from build123d import *

# Parameters (mm, degrees)
F1_DEPTH = 6.35


with BuildPart() as f1:
    # F0 (on Front) → F1 (new body)
    with BuildSketch(Plane.XZ):
        with BuildLine():
            Line((147.03905, 56.8491), (26.060874, 15.470934))
            ThreePointArc((26.060874, 15.470934), (14.468308, -7.009272), (35.415419, -21.185511))
            Line((35.415419, -21.185511), (159.893201, -17.296974))
            ThreePointArc((159.893201, -17.296974), (196.909173, 27.30746), (147.03905, 56.8491))
        make_face()
        with BuildLine():
            ThreePointArc((28.604817, 5.287778), (30.133109, 5.973494), (31.764223, 6.354742))
            Line((31.764223, 6.354742), (41.633012, -1.638817))
            ThreePointArc((41.633012, -1.638817), (40.945432, -5.75352), (38.427272, -9.079542))
            Line((38.427272, -9.079542), (28.954331, -10.074033))
            ThreePointArc((28.954331, -10.074033), (24.867546, -5.657956), (24.608037, 0.353383))
            Line((24.608037, 0.353383), (28.604817, 5.287778))
        make_face(mode=Mode.SUBTRACT)
    extrude(amount=F1_DEPTH)


solid = f1.part
Read the model definition and answer for the solid it produces. Units are mm, in the model's axes. A direction names the side the tool comes from. Give positions to 0.01 mm unless a question says otherwise; leave off trailing zeros. Write each loop counter-clockwise with the first axis right and the second up, starting at its lowest first coordinate (ties: lowest second). Pieces come first, ordered by that corner, then holes. Notation, with made-up numbers: (16, 69) - (42, 69) arc R20 ccw to (42, 91) - close; hole circle Ø4 at (55, 46.5). An arc over 180 degrees is marked (long way). Use CSV: the item, a comma, the result in double quotes. Start each with the question number.
Item 1: The mould has two halves that part along Z. Classify faces 3 (the cylindrical face through (24.901, -3.131, -5.737)), 4 (the cylindrical face through (14.376, -3.131, -6.633)), 5 (the flat face through (104, 0, 10)): pulls with the +Z half, pulls with the -Z half, needs draft (parallel to the pull), parting line crosses it, or undercut.
Item 2: The part is cut by section B-B, the plane z = -4. Give the vertices of the cut face in (x, y).
Item 3: The part is cut by section C-C, the plane x = 97.5. Give the vertices of the cut face in (y, z).
Item 4: The part is cut by section D-D, the plane z = 25. Give the vertices of the cut face in (x, y), and give its area (3 significant figures).
Item 5: Consider line 1 (X direction, y = -3.5, z = -7); line 2 (X direction, y = -4.75, z = 2); line 3 (Z direction, x = 55, y = -3). Determine where each line is inside the solid, lowest interval first.
Item 6: Flat-ended cylindrical pins translate along their axes: P1, Ø1, axis at x = 65.5, y = -5, coming from the +Z side; P2, Ø1.5, axis at x = 114, z = 21.5, coming from the +Y side. Find the tip coordinate at first contact, or state that the pin passes through.
Item 7: For faces 1 (the flat face through (36.63, -3.131, 2.414)), 2 (the flat face through (104, -6.35, 10)), determine the directions among +Z, -Z, +X, -X, +Y, -Y from which every point of the face is accessible in a straight line to the end or side of a thin tool.
Item 8: The part is cut by section A-A, the plane y = -3.5. Give the vertices of the cut face in (x, z).
Taken from the geometry:
1,face 3,"undercut"
1,face 4,"parting line crosses it"
1,face 5,"needs draft"
2,outline,"(13.95, -6.35) - (24.36, -6.35) - (24.36, 0) - (13.95, 0) - close; (41.49, -6.35) - (188.29, -6.35) - (188.29, 0) - (41.49, 0) - close"
3,outline,"(-6.35, -19.25) - (0, -19.25) - (0, 39.91) - (-6.35, 39.91) - close"
4,outline,"(53.92, -6.35) - (197.24, -6.35) - (197.24, 0) - (53.92, 0) - close"
4,area,"910 mm2"
5,line 1,"14.47 to 25.57, 40.28 to 185.42"
5,line 2,"14.37 to 25.94, 37.14 to 192.51"
5,line 3,"-20.57 to 25.37"
6,P1,"z = 29.13"
6,P2,"y = 0"
7,face 1,"+Y, -Y"
7,face 2,"+Z, -Z, +X, -X, -Y"
8,outline,"(26.06, 15.47) arc R19.05 ccw to (35.42, -21.19) - (159.89, -17.3) arc R38.1 ccw (long way) to (147.04, 56.85) - close; hole (24.61, 0.35) arc R8.73 ccw to (28.95, -10.07) - (38.43, -9.08) arc R8.73 ccw to (41.63, -1.64) - (31.76, 6.35) arc R8.73 ccw to (28.6, 5.29) - close"
